Autodesk Inventor part; units mm, degrees
ref_plane "YZ Plane" through (0, 0, 0) normal (1, 0, 0) x (0, 1, 0)
ref_plane "XZ Plane" through (0, 0, 0) normal (0, 1, 0) x (-1, 0, 0)
ref_plane "XY Plane" through (0, 0, 0) normal (0, 0, 1) x (1, 0, 0)
sketch "スケッチ1" plane through (0, 0, 0) normal (0, 0, 1) x (1, 0, 0)
  circle A0 centre (0, 0) radius 144
  arc A1 (-6.699441, 21.479467) -> (7, 21.383405) centre (0, 0) ccw
  line L0 (0, 22.5) -> (0, 17)
  line L1 (0, 22.5) -> (0, 26.3)
  line L2 (0, 26.3) -> (7, 26.3)
  line L3 (7, 26.3) -> (7, 21.383405)
  line L4 (7, 17) -> (0, 17)
  line L5 (-6.699441, 21.479467) -> (-6.699441, 26.3)
  line L6 (-6.699441, 26.3) -> (0, 26.3)
  circle A2 centre (0, 0) radius 135 construction
  circle A3 centre (0, 0) radius 131.55695 construction
  circle A4 centre (0, 0) radius 140 construction
  line L7 (0, 0) -> (139.964753, 3.141329)
  line L8 (0, 0) -> (140, 0) construction
  line L9 (0, 0) -> (134.981058, 2.261433)
  arc A5 (131.55695, 0) -> (131.538491, 2.203757) centre (0, 0) ccw
  line L10 (150.184159, 7.263201) -> (152.050707, -0.299145)
  line L11 (119.584335, 0) -> (125.15167, 0)
  circle A6 centre (0, 0) radius 131.55695 construction
  line L12 (0, 0) -> (134.981058, -2.261433)
  line L13 (150.184159, -7.263201) -> (152.050707, 0.299145)
  arc A7 (131.538491, -2.203757) -> (131.55695, 0) centre (0, 0) ccw
  line L14 (143.93152, 4.440455) -> (146.480822, 0.114106)
  line L15 (146.480822, 0.114106) -> (143.93152, -4.440455)
  line L16 (134.979291, 2.261403) -> (134.981058, 2.261433)
  line L17 (134.907008, -2.260192) -> (135.074128, -2.262992)
  line L18 (143.93152, -4.440455) -> (144.436873, -3.537595)
  line L19 (143.93152, 4.440455) -> (145.266584, 2.433754)
  line L20 (145.266584, 2.433754) -> (146.480822, 0.114106)
  line L21 (131.538491, 2.203757) -> (134.981058, 2.261433)
  line L22 (131.538491, -2.203757) -> (135.074128, -2.262992)
  line L23 (131.570586, -2.204295) -> (131.538491, -2.203757)
  arc A8 (131.538491, -2.203757) -> (131.538491, -2.203757) centre (131.538491, -2.203757) ccw
  line L24 (131.7018, 2.206493) -> (131.538491, 2.203757)
  dimension "d7" = 270
  dimension "d9" = 280
  dimension "d0" = 288
  dimension "d1" = 45
  dimension "d2" = 5.5
  dimension "d3" = 3.8
  dimension "d4" = 7
  dimension "d8" = 263.1139
  dimension "d18" = 1.28571
  dimension "d19" = 0
sketch "スケッチ1 outline for 押し出し1" plane through (0, 0, 0) normal (0, 0, 1) x (1, 0, 0)
  circle A0 centre (0, 0) radius 144
  line L0 (0, 26.3) -> (7, 26.3)
  line L1 (-6.699441, 26.3) -> (0, 26.3)
  line L2 (-6.699441, 21.479467) -> (-6.699441, 26.3)
  arc A1 (7, 21.383405) -> (-6.699441, 21.479467) centre (0, 0) cw
  line L3 (7, 26.3) -> (7, 21.383405)
extrude "押し出し1" add sketch "スケッチ1 outline for 押し出し1" along normal blind 40
sketch "スケッチ2" plane through (0, 0, 0) normal (0, 0, -1) x (-1, 0, 0)
  point P0 (0, 0)
properties part number "gear2"
Check sheet for the modelled part. Datum: model origin and axes. Units: mm. A direction names the side the tool comes from. Give positions to 0.01 mm unless a question says otherwise; leave off trailing zeros. Write each loop counter-clockwise with the first axis right and the second up, starting at its lowest first coordinate (ties: lowest second). Pieces come first, ordered by that corner, then holes.
Item 1: Cross-section at C-C (z = 25). Enter the section's corners in (x, y).
Item 2: Cross-section at D-D (x = 30). Enter the section's corners in (y, z), and give its area (3 significant figures).
Item 3: Cross-section at B-B (y = 0). Enter the section's corners in (x, z), and give its area (3 significant figures).
Item 4: Access from +Z, -Z, +X, -X, +Y, -Y to the whole of each face (thin tool, end or side, straight path). Record for faces 1 (the face through (-2, -30, 40)), 2 (the face through (0, 26.3, 20)).
Item 5: Cross-section at A-A (x = 0). Enter the section's corners in (y, z).
Item 6: Scan lines: L1, parallel to Y at x = 0, z = 9; L2, parallel to X at y = -39.5, z = 23; L3, parallel to Y at x = 42.5, z = 9. Record each from-to range of solid material in increasing order.
Item 7: Gauge pin test, flat ends, axial feed: pin 1 (3 mm diameter, centred on y = 102.5, z = 35, fed in from -X); pin 2 (6 mm diameter, centred on x = -33.5, z = 19.5, fed in from -Y); pin 3 (10 mm diameter, centred on y = -9.5, z = 18.5, fed in from -X). Record the tip position at first contact, or that the pin passes through.
Item 8: Draft check along Y on faces 3 (the face through (0.73, -22.49, 19.72)), 4 (the face through (-18.746, -142.775, 19.72)), 5 (the face through (-2, -30, 0)). Enter one of: released by +Y, released by -Y, zero draft, split by the parting line, or undercut.
Report:
1. outline: circle Ø288 at (0, 0); hole (-6.7, 21.48) arc R22.5 ccw (long way) to (7, 21.38) - (7, 26.3) - (-6.7, 26.3) - close
2. outline: (-140.84, 0) - (140.84, 0) - (140.84, 40) - (-140.84, 40) - close
2. area: 11,300 mm2
3. outline: (-144, 0) - (-22.5, 0) - (-22.5, 40) - (-144, 40) - close; (22.5, 0) - (144, 0) - (144, 40) - (22.5, 40) - close
3. area: 9,720 mm2
4. face 1: +Z, +X, -X, +Y, -Y
4. face 2: +Z, -Z
5. outline: (-144, 0) - (-22.5, 0) - (-22.5, 40) - (-144, 40) - close; (26.3, 0) - (144, 0) - (144, 40) - (26.3, 40) - close
6. L1: y = -144 to -22.5, 26.3 to 144
6. L2: x = -138.48 to 138.48
6. L3: y = -137.59 to 137.59
7. pin 1: stops at x = -102.64
7. pin 2: stops at y = -140.73
7. pin 3: stops at x = -143.93
8. face 3: undercut
8. face 4: split by the parting line
8. face 5: zero draft
